Input: part model. Units: mm. Frame: model coordinates. Coordinates: 2 decimals unless noted, no trailing zeros. Loops run counter-clockwise (first coordinate to the right, second up) from the corner with the lowest first, then second, coordinate; pieces in that order, holes last. Notation, with made-up numbers: (62.5, 67.25) - (66.5, 67.25) arc R28 cw to (66.5, 103.25) - close; hole circle Ø5 at (21.5, 18.25). An arc over 180 degrees is marked (long way). Use a Markdown table: item, result. Add a question column.
1. Section query B-B on y = 4. Return the cut outline in (x, z), then the cut area to 3 significant figures.
2. Draft query along Z for faces 1 (the face through (-4, 0, -13)), 2 (the face through (-2.38, 3.22, 10.74)). Return one class per face: released by +Z, released by -Z, zero draft, split by the parting line, or undercut.
3. Section query A-A on x = 0. Return the cut outline in (y, z), then the cut area to 3 significant figures.
4. Contact query for flat-ended pins moving along their axis: P1, Ø5, axis at x = 279.4, z = 0, coming from the -Y side; P2, Ø4, axis at x = -91.5, z = 7.5, coming from the -Y side. Output: stop coordinate, or through.
5. Ray query, L1, parallel to Z at x = 279.4, y = 1.5; L2, parallel to X at y = 3, z = -2.5; L3, parallel to Z at x = 0, y = 5. Return the intervals inside material, ascending. Write a range as [from, to].
```python
from build123d import *

# Parameters (mm, degrees)
SKETCH1_W                = 609.6
SKETCH1_H                = 38.1
BOSS_EXTRUDE1_DEPTH      = 6.35
SKETCH2_R                = 11
CUT_EXTRUDE1_DEPTH       = 7.62
F_0_257_DIAMETER_HOLE2_D = 6.5278


with BuildPart() as part:
    # Sketch1 → Boss-Extrude1 (new body)
    with BuildSketch(Plane(origin=(0, 0, 0), x_dir=(1, 0, 0), z_dir=(0, 1, 0))):
        Rectangle(SKETCH1_W, SKETCH1_H)
    extrude(amount=BOSS_EXTRUDE1_DEPTH)

    # Sketch2 → Cut-Extrude1 (cut)
    with BuildSketch(Plane(origin=(0, 6.35, 0), x_dir=(1, 0, 0), z_dir=(0, 1, 0))):
        Circle(SKETCH2_R)
    extrude(amount=-CUT_EXTRUDE1_DEPTH, mode=Mode.SUBTRACT)

    # F (0.257) Diameter Hole2 (through all)
    with Locations(Plane(origin=(0, 6.35, 0), x_dir=(1, 0, 0), z_dir=(0, 1, 0))):
        with Locations((-241.3, 0), (-279.4, 0)):
            f_0_257_diameter_hole2 = Hole(F_0_257_DIAMETER_HOLE2_D / 2)

    # Mirror1: F (0.257) Diameter Hole2 across plane
    add(f_0_257_diameter_hole2.mirror(Plane(origin=(0, 0, 0), x_dir=(0, 0, 1), z_dir=(1, 0, 0))), mode=Mode.SUBTRACT)


solid = part.part
```
Resolved:
| question | item | result |
|---|---|---|
| 1 | outline | (-304.8, -19.05) - (304.8, -19.05) - (304.8, 19.05) - (-304.8, 19.05) - close; hole circle Ø6.53 at (-279.4, 0); hole circle Ø6.53 at (-241.3, 0); hole circle Ø22 at (0, 0); hole circle Ø6.53 at (241.3, 0); hole circle Ø6.53 at (279.4, 0) |
| 1 | area | 22,700 mm² |
| 2 | face 1 | zero draft |
| 2 | face 2 | undercut |
| 3 | outline | (0, -19.05) - (6.35, -19.05) - (6.35, -11) - (0, -11) - close; (0, 11) - (6.35, 11) - (6.35, 19.05) - (0, 19.05) - close |
| 3 | area | 102 mm² |
| 4 | P1 | through |
| 4 | P2 | y = 0 |
| 5 | L1 | [-19.05, -3.26], [3.26, 19.05] |
| 5 | L2 | [-304.8, -281.5], [-277.3, -243.4], [-239.2, -10.71], [10.71, 239.2], [243.4, 277.3], [281.5, 304.8] |
| 5 | L3 | [-19.05, -11], [11, 19.05] |
